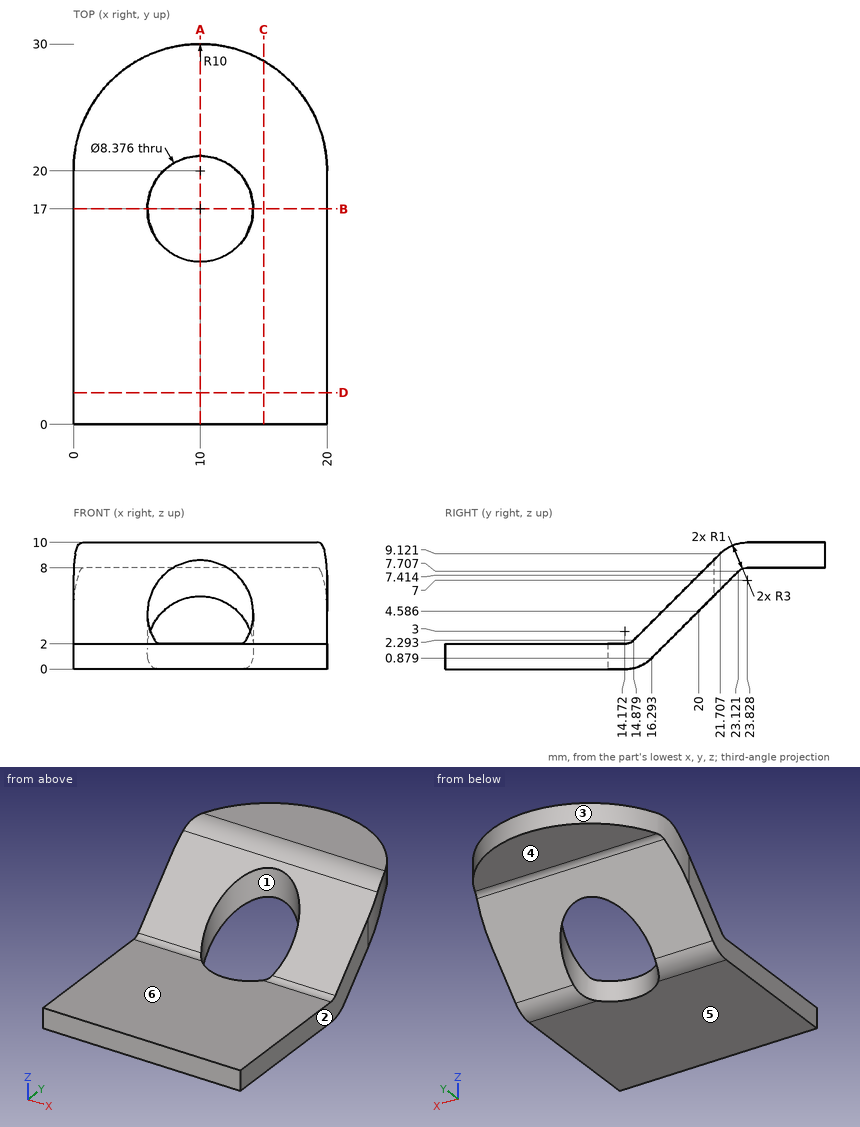
Part print with two shaded views. Sizes in mm from the minimum x, y, z corner. A direction names the side the tool comes from. Give positions to 0.01 mm unless a question says otherwise; leave off trailing zeros. Order: outer loops, then holes, each group sorted by start corner. A loop starts at its lowest first (then second) coordinate and runs counter-clockwise, first axis right, second up.
(1) Drill centre lines: L1, parallel to X at y = 17, z = 2.5; L2, parallel to Z at x = 3.5, y = 10.5; L3, parallel to Z at x = 12.25, y = 29. Where is each one in solid material? Low to high.
(2) Saw through at C-C, the plane x = 15. Give the cut face in (y, z).
(3) Mould opens along Y. For the marked faces 1, 2 and 3 say: released by +Y, released by -Y, zero draft, split by the parting line, or undercut.
(4) Tool access for the marked faces 4, 5 and 6: list every direction of +Z, -Z, +X, -X, +Y, -Y with a clear straight run to the whole face (end or side of a thin tool).
(5) Saw through at B-B, the plane y = 17. Give the cut face in (x, z).
(6) Saw through at D-D, the plane y = 2.5. Give the cut face in (x, z), then the cut area to 3 significant figures.
(7) Saw through at A-A, the plane x = 10. Give the cut face in (y, z).
(8) Flat gauge pins, fed straight in: pin 1 (1 mm diameter, centred on x = 7, y = 14.5, fed in from +Z); pin 2 (1.5 mm diameter, centred on x = 14, z = 9, fed in from -Y) (1 decimal); pin 3 (2 mm diameter, centred on x = 7.5, z = 7, fed in from -Y) (1 decimal); pin 4 (7.5 mm diameter, centred on x = 10, y = 17, fed in from +Z). Where does each tip first touch, or does it go through?
Results found:
1. L1: x = 0 to 5.81, 14.19 to 20
1. L2: z = 0 to 2
1. L3: z = 8 to 10
2. outline: (0, 0) - (14.17, 0) arc R3 ccw to (16.29, 0.88) - (23.12, 7.71) arc R1 cw to (23.83, 8) - (28.66, 8) - (28.66, 10) - (23.83, 10) arc R3 ccw to (21.71, 9.12) - (14.88, 2.29) arc R1 cw to (14.17, 2) - (0, 2) - close
3. face 1: undercut
3. face 2: zero draft
3. face 3: released by +Y
4. face 4: -Z, +X, -X, +Y
4. face 5: -Z, +X, -X, +Y, -Y
4. face 6: +Z, +X, -X, -Y
5. outline: (0, 1.59) - (5.81, 1.59) - (5.81, 4.41) - (0, 4.41) - close; (14.19, 1.59) - (20, 1.59) - (20, 4.41) - (14.19, 4.41) - close
6. outline: (0, 0) - (20, 0) - (20, 2) - (0, 2) - close
6. area: 40.0 mm2
7. outline: (0, 0) - (12.81, 0) - (12.81, 2) - (0, 2) - close; (21.19, 5.77) - (23.12, 7.71) arc R1 cw to (23.83, 8) - (30, 8) - (30, 10) - (23.83, 10) arc R3 ccw to (21.71, 9.12) - (21.19, 8.6) - close
8. pin 1: stops at z = 2.13
8. pin 2: stops at y = 20.8
8. pin 3: stops at y = 19.3
8. pin 4: passes through
